Part model, mm, in its own coordinate system. A direction names the side the tool comes from. Coordinates: 2 decimals unless noted, no trailing zeros. Loops run counter-clockwise (first coordinate to the right, second up) from the corner with the lowest first, then second, coordinate; pieces in that order, holes last. Notation, with made-up numbers: (47, 24.5) -> (70, 24.5) arc R31 cw to (70, 63.5) -> close; hole circle Ø4 at (32, -31). An arc over 180 degrees is marked (long way). Use one line per item in the form item = value. Start each with the question number.
(1) Band-saw the part on A-A on z = 13. Give the cut face in (x, y).
(2) Band-saw the part on D-D on x = -71.5. Give the cut face in (y, z), then the cut area to 3 significant figures.
(3) Band-saw the part on B-B on y = -4. Count the separate pieces of the cut face and the enclosed holes in it, then the cut area to 3 significant figures.
(4) Pin check, flat tips, straight feed: P1, Ø17, axis at y = -18.5, z = 13.5, coming from the -X side; P2, Ø4, axis at x = 14, z = 12, coming from the +Y side; P3, Ø5, axis at y = 47.5, z = 17.5, coming from the -X side; P4, Ø5, axis at x = 7.5, y = -5, coming from the -Z side. Stop position of each tip, or through.
(5) Drill centre lines: L1, parallel to X at y = 12, z = 9; L2, parallel to X at y = 23, z = 18.5; L3, parallel to Z at x = -34, y = 40. Where is each one in solid material? Low to high. Write a range as [from, to].
(6) 3-axis set-ups, long thin cutter, end or side, ignore diameter. For faces 1 (the cylindrical face through (27.14, 26.31, 12.4)), 2 (the flat face through (13.55, 1.057, 7.363)), 3 (the flat face through (-62.011, -17, 12)): which of +Z, -Z, +X, -X, +Y, -Y reach the whole face in a straight line?
(7) Mould opens along Z. For faces 4 (the flat face through (-1, -25, 6)), 5 (the flat face through (-40.862, 14.065, 17.637)), 6 (the flat face through (-26.708, 5.357, 17.488)), 7 (the cylindrical face through (1, -23, 24)) say: +Z half, -Z half, draft (parallel to the pull), parting line (faces both ways), or undercut.
(8) Band-saw the part on C-C on y = 43. Give the cut face in (x, z).
```python
from build123d import *

# Parameters (mm, degrees)
F1_DEPTH      = 25
F2_DEPTH      = 40
F2_DEPTH_BACK = 20
F4_DEPTH      = 84.4041628775
F5_R          = 5


with BuildPart() as f1:
    # F0 (on Top) → F1 (new body)
    with BuildSketch(Plane.XY):
        with BuildLine():
            Line((-62.0106605823, -25), (62.0106605823, -25))
            Line((62.0106605823, -25), (62.0106605823, 25))
            Line((62.0106605823, 25), (-27.6074977048, 25))
            ThreePointArc((-27.6074977048, 25), (-37.6839508173, 0.6732902351), (-62.0106605823, -9.4031628775))
            Line((-62.0106605823, -9.4031628775), (-62.0106605823, -25))
        make_face()
        with BuildLine():
            Line((-27.6074977048, 25), (62.0106605823, 25))
            ThreePointArc((62.0106605823, 25), (16.3862035085, 27.2471495314), (-28.7966079142, 33.9668456737))
            ThreePointArc((-28.7966079142, 33.9668456737), (-27.9060708638, 29.5226735573), (-27.6074977048, 25))
        make_face()
        with BuildLine():
            ThreePointArc((-28.7966079142, 33.9668456737), (-89.3242603833, 45.9175735181), (-62.0106605823, -9.4031628775))
            Line((-62.0106605823, -9.4031628775), (-62.0106605823, 8.7209436981))
            ThreePointArc((-62.0106605823, 8.7209436981), (-78.1512656311, 27.1186181204), (-57.8094614837, 40.7276063092))
            ThreePointArc((-57.8094614837, 40.7276063092), (-43.3572727982, 37.1144708153), (-28.7966079142, 33.9668456737))
        make_face()
        with BuildLine():
            Line((-62.0106605823, 8.7209436981), (-62.0106605823, -9.4031628775))
            ThreePointArc((-62.0106605823, -9.4031628775), (-37.6839508173, 0.6732902351), (-27.6074977048, 25))
            Line((-27.6074977048, 25), (-45.7316042803, 25))
            ThreePointArc((-45.7316042803, 25), (-50.4996294799, 13.4889688976), (-62.0106605823, 8.7209436981))
        make_face()
        with BuildLine():
            Line((-45.7316042803, 25), (-27.6074977048, 25))
            ThreePointArc((-27.6074977048, 25), (-27.9060708638, 29.5226735573), (-28.7966079142, 33.9668456737))
            ThreePointArc((-28.7966079142, 33.9668456737), (-43.3572727982, 37.1144708153), (-57.8094614837, 40.7276063092))
            ThreePointArc((-57.8094614837, 40.7276063092), (-49.0994400601, 34.9150420428), (-45.7316042803, 25))
        make_face()
    extrude(amount=F1_DEPTH)

    # F0 (on Top) → F2 (join, two sides)
    with BuildSketch(Plane.XY) as f2_sk:
        with BuildLine():
            ThreePointArc((-57.8094614837, 40.7276063092), (-78.1512656311, 27.1186181204), (-62.0106605823, 8.7209436981))
            Line((-62.0106605823, 8.7209436981), (-62.0106605823, 25))
            Line((-62.0106605823, 25), (-45.7316042803, 25))
            ThreePointArc((-45.7316042803, 25), (-49.0994400601, 34.9150420428), (-57.8094614837, 40.7276063092))
        make_face()
        with BuildLine():
            Line((-62.0106605823, 25), (-62.0106605823, 8.7209436981))
            ThreePointArc((-62.0106605823, 8.7209436981), (-50.4996294799, 13.4889688976), (-45.7316042803, 25))
            Line((-45.7316042803, 25), (-62.0106605823, 25))
        make_face()
    extrude(amount=F2_DEPTH)
    extrude(f2_sk.sketch, amount=-F2_DEPTH_BACK)

    # F3 (on face) → F4 (cut, through all)
    with BuildSketch(Plane.XZ.offset(25)):
        Polygon((-43.4297714291, 5.7516291939), (-37.6987736764, 9.3219915203), (-37.9252992754, 16.0703623264), (-43.882822627, 19.2483708061), (-49.6138203798, 15.6780084797), (-49.3872947808, 8.9296376736), align=None)
        Polygon((-23.882822627, 19.2483708061), (-29.6138203798, 15.6780084797), (-29.3872947808, 8.9296376736), (-23.4297714291, 5.7516291939), (-17.6987736764, 9.3219915203), (-17.9252992754, 16.0703623264), align=None)
        Polygon((-3.882822627, 19.2483708061), (-9.6138203798, 15.6780084797), (-9.3872947808, 8.9296376736), (-3.4297714291, 5.7516291939), (2.3012263236, 9.3219915203), (2.0747007246, 16.0703623264), align=None)
        Polygon((16.117177373, 19.2483708061), (10.3861796202, 15.6780084797), (10.6127052192, 8.9296376736), (16.5702285709, 5.7516291939), (22.3012263236, 9.3219915203), (22.0747007246, 16.0703623264), align=None)
        Polygon((36.117177373, 19.2483708061), (30.3861796202, 15.6780084797), (30.6127052192, 8.9296376736), (36.5702285709, 5.7516291939), (42.3012263236, 9.3219915203), (42.0747007246, 16.0703623264), align=None)
    extrude(amount=-F4_DEPTH, mode=Mode.SUBTRACT)

    # F5
    f5_edges = [f1.edges().sort_by_distance(p)[0] for p in [
        (0, -25, 25),
        (0, -25, 0),
        (16.386204, 27.24715, 0),
        (16.386204, 27.24715, 25),
    ]]
    fillet(f5_edges, radius=F5_R)


solid = f1.part
```
A:
q1.outline = (-62.01, -25) -> (-49.52, -25) -> (-49.52, 57.06) arc R34.4 ccw (long way) to (-62.01, -9.4) -> close; (-37.82, -25) -> (-29.52, -25) -> (-29.52, 36.32) arc R34.4 ccw to (-37.82, 49.46) -> close; (-17.82, -25) -> (-9.52, -25) -> (-9.52, 30.54) arc R464.29 cw to (-17.82, 31.92) -> close; (2.18, -25) -> (10.48, -25) -> (10.48, 27.87) arc R464.29 cw to (2.18, 28.87) -> close; (22.18, -25) -> (30.48, -25) -> (30.48, 26.07) arc R464.29 cw to (22.18, 26.71) -> close; (42.18, -25) -> (62.01, -25) -> (62.01, 25) arc R464.29 cw to (42.18, 25.42) -> close
q2.outline = (-8.07, 0) -> (11.77, 0) -> (11.77, -20) -> (38.23, -20) -> (38.23, 0) -> (58.07, 0) -> (58.07, 25) -> (38.23, 25) -> (38.23, 40) -> (11.77, 40) -> (11.77, 25) -> (-8.07, 25) -> close
q2.area = 2,580 mm²
q3.separate_pieces = 1
q3.enclosed_holes = 5
q3.area = 2,970 mm²
q4.P1 = -62.01
q4.P2 = through
q4.P3 = -90
q4.P4 = 0
q5.L1 = [-93.86, -49.39], [-38.22, -29.39], [-18.22, -9.39], [1.78, 10.61], [21.78, 30.61], [41.78, 62.01]
q5.L2 = [-96.36, -45.08], [-42.48, -25.08], [-22.48, -5.08], [-2.48, 14.92], [17.52, 34.92], [37.52, 62.01]
q5.L3 = [0, 25]
q6.face_1 = +Z, -Z, +X, +Y
q6.face_2 = +Y, -Y
q6.face_3 = +Z, -Z, -X, -Y
q7.face_4 = draft
q7.face_5 = undercut
q7.face_6 = undercut
q7.face_7 = +Z half
q8.outline = (-91.33, 0) -> (-32.69, 0) -> (-32.69, 25) -> (-91.33, 25) -> close; hole (-49.61, 15.68) -> (-49.39, 8.93) -> (-43.43, 5.75) -> (-37.7, 9.32) -> (-37.93, 16.07) -> (-43.88, 19.25) -> close
